Can you work these out from the drawing? Everything is in mm from the part's minimum corner. Coordinates: 2 decimals unless noted, no trailing zeros. Order: outer loops, then holes, each group sorted by start corner. A loop starts at its lowest first (then second) coordinate and runs counter-clockwise, first axis right, second up. Notation, with made-up numbers: (14, 14) - (36, 14) arc R12 cw to (36, 19) - close; hole circle Ø5 at (3, 3). An arc over 180 degrees is marked (long way). Use a Markdown table: item, result. Add a question column.
(1) I want a section at B-B (x = 40). List the corners of the cut face in (y, z) for me.
(2) I want a section at A-A (y = 4.5). List the corners of the cut face in (x, z) for me.
(3) I want a section at C-C (z = 1.5). List the corners of the cut face in (x, y) for me, and give its area (3 significant figures).
(4) If I drill on L1, parallel to Y at x = 25.5, z = 3.25 (3 decimals); L2, parallel to X at y = 40, z = 18.5; L3, parallel to X at y = 45, z = 5, over which ranges is the centre line in solid material (lowest first)? Write a range as [from, to].
(5) I want a section at D-D (y = 28.5). List the corners of the cut face in (x, z) for me.
(6) We'd pull the mould along Y, two halves only. Please class the marked faces 1 and 2: pulls with the +Y half, pulls with the -Y half, needs draft (parallel to the pull), parting line crosses it, or undercut.
(7) For pin 1 Ø8 at (y, z) = (10.5, 13.5) entering from +X; pin 2 Ø10 at (y, z) = (21, 4.5) entering from +X; pin 3 Ø6 at (y, z) = (36, 7) entering from +X; pin 4 Ø6 at (y, z) = (35, 9) entering from +X, each with a flat end and sliding along its axis, tell me the tip position at first contact or that it passes through.
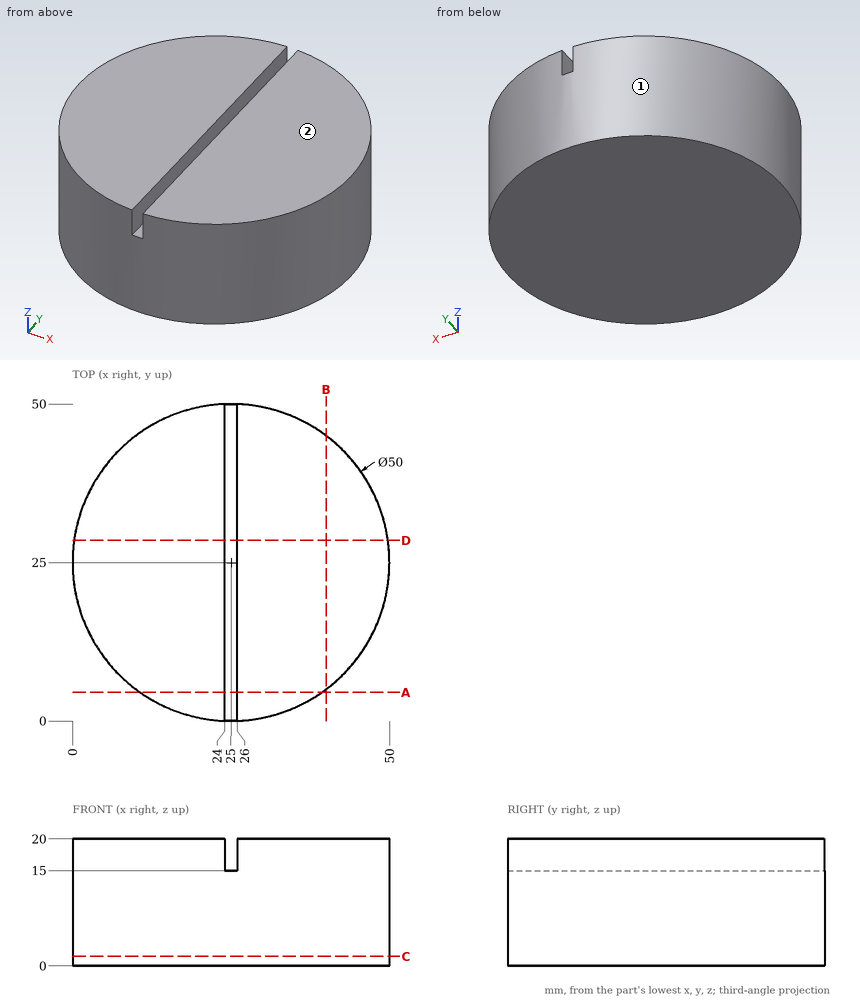
Answers follow:
| question | item | result |
|---|---|---|
| 1 | outline | (5, 0) - (45, 0) - (45, 20) - (5, 20) - close |
| 2 | outline | (10.69, 0) - (39.31, 0) - (39.31, 20) - (26, 20) - (26, 15) - (24, 15) - (24, 20) - (10.69, 20) - close |
| 3 | outline | circle Ø50 at (25, 25) |
| 3 | area | 1,960 mm² |
| 4 | L1 | y = [0.005, 49.995] |
| 4 | L2 | x = [5, 24], [26, 45] |
| 4 | L3 | x = [10, 40] |
| 5 | outline | (0.25, 0) - (49.75, 0) - (49.75, 20) - (26, 20) - (26, 15) - (24, 15) - (24, 20) - (0.25, 20) - close |
| 6 | face 1 | parting line crosses it |
| 6 | face 2 | needs draft |
| 7 | pin 1 | stops at x = 47.69 |
| 7 | pin 2 | stops at x = 50 |
| 7 | pin 3 | stops at x = 48.69 |
| 7 | pin 4 | stops at x = 49 |
